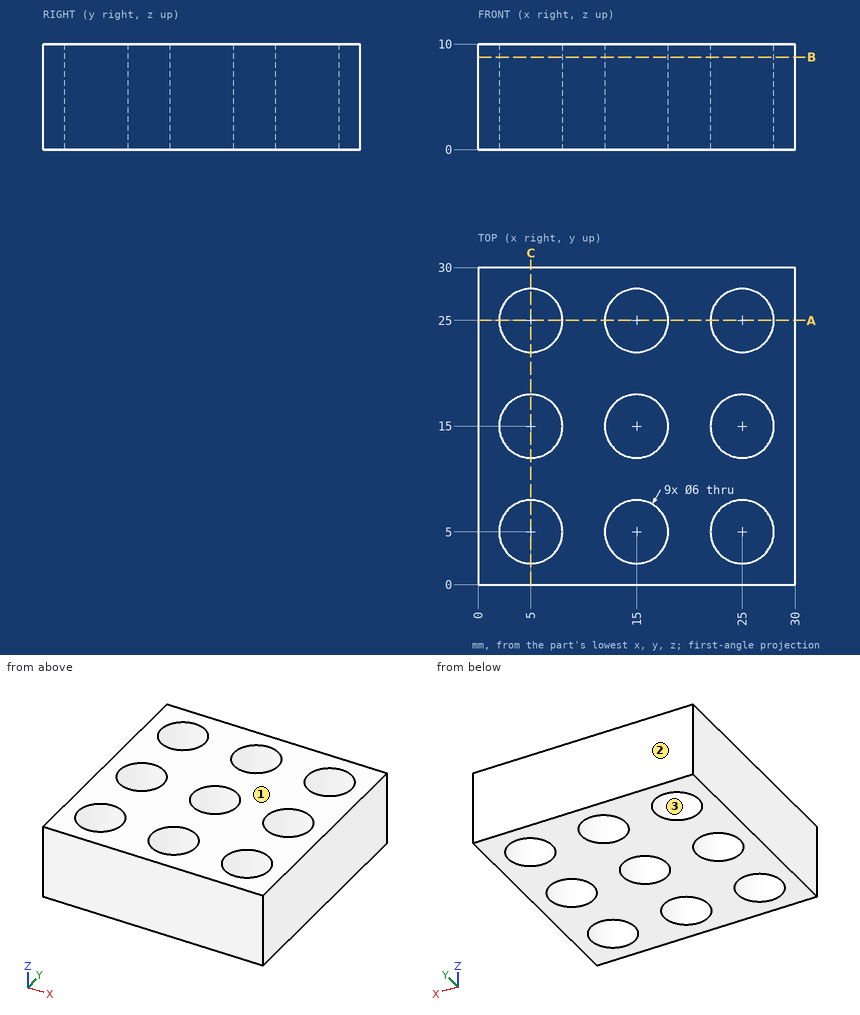
The figure shows three views and two pictorial views of one solid part (mm, origin at its lowest corner). Answer the questions. Coordinates: 2 decimals unless noted, no trailing zeros. Loops run counter-clockwise (first coordinate to the right, second up) from the corner with the lowest first, then second, coordinate; pieces in that order, holes last. Notation, with made-up numbers: M -20.75,42.25 L 13.25,42.25 A13 ccw 13.25,63.25 Z; hole C -28,-25.75 d1. An arc over 180 degrees is marked long. Answer as CSV lines item,"result". Start each with the question number.
(1) Find the intervals of material crossed by L1, parallel to Y at x = 15, z = 4.5; L2, parallel to Y at x = 26, z = 8; L3, parallel to X at y = 26.25, z = 8.25, in increasing order. Write a range as [from, to].
(2) The part is cut by section B-B (z = 8.75). State how many separate pieces and enclosed holes the cut face has, and give its area (3 significant figures).
(3) The part is cut by section A-A (y = 25). Give the vertices of the cut face in (x, z).
(4) The mould has two halves that part along Y. Classify the marked faces 1, 2 and 3: pulls with the +Y half, pulls with the -Y half, needs draft (parallel to the pull), parting line crosses it, or undercut.
Determined:
1,L1,"[0, 2], [8, 12], [18, 22], [28, 30]"
1,L2,"[0, 2.17], [7.83, 12.17], [17.83, 22.17], [27.83, 30]"
1,L3,"[0, 2.27], [7.73, 12.27], [17.73, 22.27], [27.73, 30]"
2,separate pieces,"1"
2,enclosed holes,"9"
2,area,"646 mm2"
3,outline,"M 0,0 L 2,0 L 2,10 L 0,10 Z; M 8,0 L 12,0 L 12,10 L 8,10 Z; M 18,0 L 22,0 L 22,10 L 18,10 Z; M 28,0 L 30,0 L 30,10 L 28,10 Z"
4,face 1,"needs draft"
4,face 2,"pulls with the +Y half"
4,face 3,"undercut"
